For this review, use the dimensioned drawing (mm, ordinates from the lowest corner) and the shaded views. Coordinates: 2 decimals unless noted, no trailing zeros. Loops run counter-clockwise (first coordinate to the right, second up) from the corner with the lowest first, then second, coordinate; pieces in that order, holes last. Notation, with made-up numbers: (52, 8.25) -> (72, 8.25) arc R32 cw to (72, 38.25) -> close; hole circle Ø9 at (77, 31). An arc over 180 degrees is marked (long way). One line per question, with ' | ' between items. Start each with the question number.
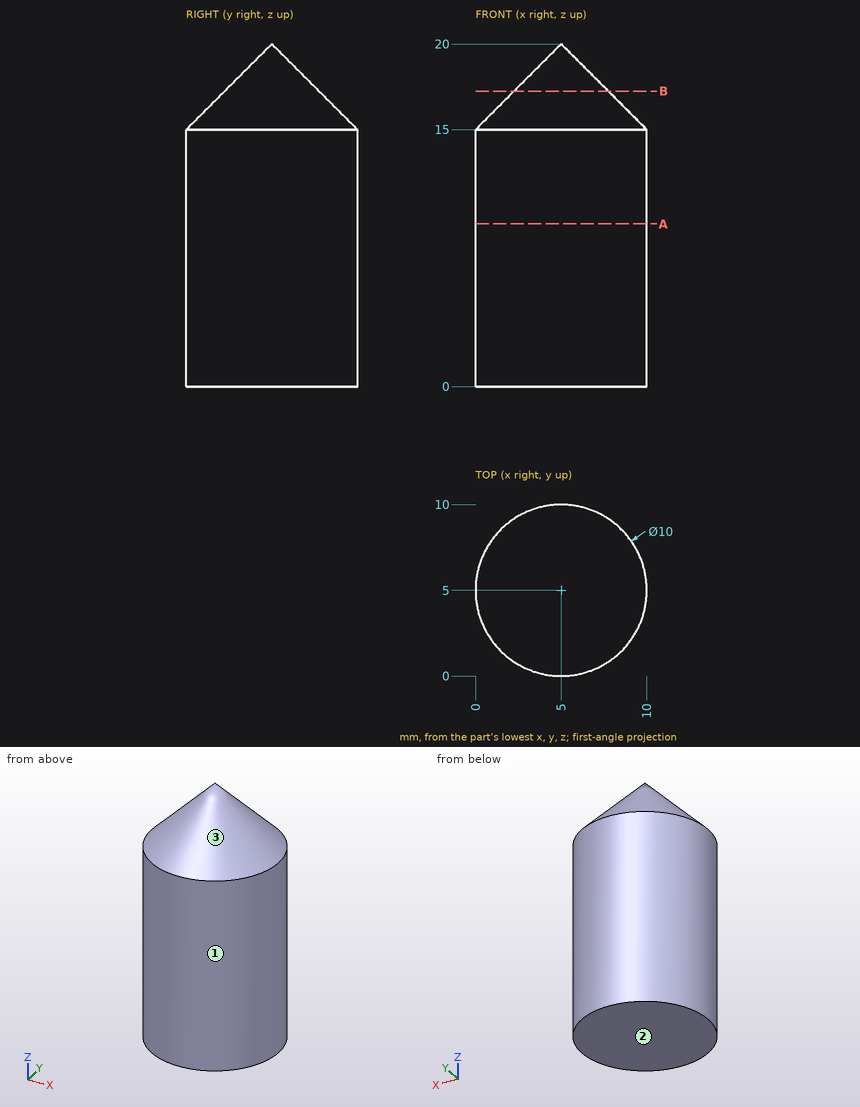
1) Wall thickness on L1, parallel to Z at x = 2.5, y = 8.5; L2, parallel to Z at x = 4.25, y = 8.25; L3, parallel to Y at x = 3.25, z = 13.25: over which ranges is each line inside the solid? List them lowest first.
2) Consider section B-B, the plane z = 17.25. Write out the cut boundary in (x, y).
3) Consider section A-A, the plane z = 9.5. Write out the cut boundary in (x, y), plus the area to 3 significant figures.
4) Mouldability with a two-part tool opening along Z and no side actions: class the marked faces 1, 2 and 3 as +Z half, -Z half, draft (parallel to the pull), parting line (faces both ways), or undercut.
5) Insertion check: pin 1 Ø2 at (x, y) = (6.5, 8) entering from +Z; pin 2 Ø3 at (y, z) = (2, 11.5) entering from +X; pin 3 Ø4 at (x, z) = (2.5, 10.5) entering from -Y. Each pin has a flat end and moves straight along its axis. Give the tip position at first contact, or say it passes through.
Filled sheet:
1) L1: 0 to 15.7 | L2: 0 to 16.66 | L3: 0.32 to 9.68
2) outline: circle Ø5.5 at (5, 5)
3) outline: circle Ø10 at (5, 5) | area: 78.5 mm^2
4) face 1: draft | face 2: -Z half | face 3: +Z half
5) pin 1: z = 17.65 | pin 2: x = 9.77 | pin 3: y = 0.03
